Part model, mm, in its own coordinate system. A direction names the side the tool comes from. Give positions to 0.01 mm unless a question says otherwise; leave off trailing zeros. Write each loop counter-clockwise with the first axis right and the second up, starting at its lowest first coordinate (ties: lowest second). Pieces come first, ordered by that corner, then holes.
```python
from build123d import *

# Parameters (mm, degrees)
SKETCH1_W               = 25.4
SKETCH1_H               = 22.86
BOSS_EXTRUDE1_DEPTH     = 5.4864
SKETCH2_R               = 2.5
SKETCH2_R_2             = 1.25
BOSS_EXTRUDE2_DEPTH     = 11
SKETCH5_R               = 1.25
CUT_EXTRUDE1_DEPTH      = 1
CUT_EXTRUDE1_DEPTH_BACK = 17.4864


with BuildPart() as part:
    # Sketch1 → Boss-Extrude1 (new body)
    with BuildSketch(Plane(origin=(0, 0, 0), x_dir=(1, 0, 0), z_dir=(0, 1, 0))):
        with Locations((-21.340699551, -9.756889686)):
            Rectangle(SKETCH1_W, SKETCH1_H)
    extrude(amount=BOSS_EXTRUDE1_DEPTH)

    # Sketch2 → Boss-Extrude2 (add)
    with BuildSketch(Plane.XZ):
        with Locations((-31.918497565, 18.367860399)):
            Circle(SKETCH2_R)
        with Locations((-31.918497565, 18.367860399)):
            Circle(SKETCH2_R_2, mode=Mode.SUBTRACT)
        with Locations((-31.918497565, 0.511660399)):
            Circle(SKETCH2_R)
        with Locations((-31.918497565, 0.511660399)):
            Circle(SKETCH2_R_2, mode=Mode.SUBTRACT)
        with Locations((-11.420697565, 0.511660399)):
            Circle(SKETCH2_R)
        with Locations((-11.420697565, 0.511660399)):
            Circle(SKETCH2_R_2, mode=Mode.SUBTRACT)
        with Locations((-11.420697565, 18.367860399)):
            Circle(SKETCH2_R)
        with Locations((-11.420697565, 18.367860399)):
            Circle(SKETCH2_R_2, mode=Mode.SUBTRACT)
    extrude(amount=BOSS_EXTRUDE2_DEPTH)

    # Sketch5 → Cut-Extrude1 (cut, two sides)
    with BuildSketch(Plane(origin=(0, 5.4864, 0), x_dir=(1, 0, 0), z_dir=(0, 1, 0))) as cut_extrude1_sk:
        with Locations((-31.918497565, -0.511660399)):
            Circle(SKETCH5_R)
        with Locations((-11.420697565, -0.511660399)):
            Circle(SKETCH5_R)
        with Locations((-11.420697565, -18.367860399)):
            Circle(SKETCH5_R)
        with Locations((-31.918497565, -18.367860399)):
            Circle(SKETCH5_R)
    extrude(amount=CUT_EXTRUDE1_DEPTH, mode=Mode.SUBTRACT)
    extrude(cut_extrude1_sk.sketch, amount=-CUT_EXTRUDE1_DEPTH_BACK, mode=Mode.SUBTRACT)


solid = part.part
```
1) Saw through at D-D, the plane z = 16.5. Write the cut outline in (x, y), then the cut area to 3 significant figures.
Answers follow:
outline: (-34.04, 0) - (-33.58, 0) - (-33.58, -11) - (-30.26, -11) - (-30.26, 0) - (-13.08, 0) - (-13.08, -11) - (-9.76, -11) - (-9.76, 0) - (-8.64, 0) - (-8.64, 5.49) - (-34.04, 5.49) - close
area: 212 mm2
2) Saw through at C-C, the plane y = 2.75. Write the cut outline in (x, z).
Answers follow:
outline: (-34.04, -1.67) - (-8.64, -1.67) - (-8.64, 21.19) - (-34.04, 21.19) - close; hole circle Ø2.5 at (-31.92, 0.51); hole circle Ø2.5 at (-31.92, 18.37); hole circle Ø2.5 at (-11.42, 0.51); hole circle Ø2.5 at (-11.42, 18.37)
3) Saw through at B-B, the plane x = -30. Write the cut outline in (y, z).
Answers follow:
outline: (-11, -1.09) - (0, -1.09) - (0, -1.67) - (5.49, -1.67) - (5.49, 21.19) - (0, 21.19) - (0, 19.97) - (-11, 19.97) - (-11, 16.76) - (0, 16.76) - (0, 2.11) - (-11, 2.11) - close
4) Wall check: L1, parallel to X at y = -9.25, z = 0.5; L2, parallel to X at y = 2.75, z = 18.5; L3, parallel to Y at x = -16.5, z = 20. Give the ranges that are in metal, low to high.
Answers follow:
L1: x = -34.42 to -33.17, -30.67 to -29.42, -13.92 to -12.67, -10.17 to -8.92
L2: x = -34.04 to -33.16, -30.68 to -12.66, -10.18 to -8.64
L3: y = 0 to 5.49
5) Saw through at A-A, the plane y = -0.5. Write the cut outline in (x, z), then the cut area to 3 significant figures.
Answers follow:
outline: circle Ø5 at (-31.92, 0.51); circle Ø5 at (-31.92, 18.37); circle Ø5 at (-11.42, 0.51); circle Ø5 at (-11.42, 18.37); hole circle Ø2.5 at (-31.92, 0.51); hole circle Ø2.5 at (-31.92, 18.37); hole circle Ø2.5 at (-11.42, 0.51); hole circle Ø2.5 at (-11.42, 18.37)
area: 58.9 mm2
6) Two-plate mould, pull along X, no slides. Class faces 6 (the face through (-11, -11, 20)), 7 (the face through (-34.041, 3, 10)), 8 (the face through (-10.228, -2.641, 0.136)), 9 (the face through (-8.641, 3, 10)): +X half, -X half, draft (parallel to the pull), parting line (faces both ways), or undercut.
Answers follow:
face 6: draft
face 7: -X half
face 8: undercut
face 9: +X half
7) 3-axis set-ups, long thin cutter, end or side, ignore diameter. For faces 1 (the face through (-31, -11, 20)), 2 (the face through (-33.8, 0, -1.4)), 3 (the face through (-33.167, -2.641, 0.457)), 4 (the face through (-22, 0, 10)), 5 (the face through (-22, 3, -1.673)): which of +Z, -Z, +X, -X, +Y, -Y reach the whole face in a straight line?
Answers follow:
face 1: +Z, -Z, +X, -X, -Y
face 2: -Z, -X, -Y
face 3: +Y, -Y
face 4: -Y
face 5: -Z, +X, -X, +Y
8) Pin check, flat tips, straight feed: pin 1 Ø2.5 at (y, z) = (2, 10.5) entering from -X; pin 2 Ø2 at (x, z) = (-11.42, 18.37) entering from -Y; pin 3 Ø2.5 at (x, y) = (-16.5, 2) entering from -Z; pin 4 Ø11.5 at (x, z) = (-26, 7.5) entering from -Y. Stop position of each tip, or through.
Answers follow:
pin 1: stops at x = -34.04
pin 2: passes through
pin 3: stops at z = -1.67
pin 4: stops at y = 0
